from build123d import *

# Parameters (mm, degrees)
MAINBASESKETCH_W         = 7.9
MAINBASESKETCH_H         = 3.2
MAINBASEEXTRUDE_DEPTH    = 7.9
MAINBASESHELL_T          = -1.2
SKETCH171_W              = 5.5
SKETCH171_H              = 1.191135725
BOSS_EXTRUDE23_DEPTH     = 2
CUT_EXTRUDE58_DEPTH      = 12.83470157
CUT_EXTRUDE58_DEPTH_BACK = 12.83470157
SWEEP28_DEPTH            = 3.2
PLAINHALF3_DEPTH         = 2
CUT_EXTRUDE59_DEPTH      = 13.162994561


# Read off the part's stored shape, not the designer's step: Sweep28
with BuildPart() as part:
    # MainBaseSketch → MainBaseExtrude (new, symmetric)
    with BuildSketch(Plane.XY):
        with Locations((4.631967213, 1.6)):
            Rectangle(MAINBASESKETCH_W, MAINBASESKETCH_H)
    extrude(amount=MAINBASEEXTRUDE_DEPTH, both=True)

    # MainBaseShell
    mainbaseshell_openings = [part.faces().sort_by_distance(p)[0] for p in [
        (4.631967213, 0, 0),
    ]]
    offset(amount=MAINBASESHELL_T, openings=mainbaseshell_openings, kind=Kind.INTERSECTION)

    # Sketch171 → Boss-Extrude23 (add)
    with BuildSketch(Plane(origin=(0, 2, 0), x_dir=(-1, 0, 0), z_dir=(0, -1, 0))):
        with Locations((-4.631967213, -0.595567863)):
            Rectangle(SKETCH171_W, SKETCH171_H)
    extrude(amount=BOSS_EXTRUDE23_DEPTH)

    # Sketch173 → Cut-Extrude58 (cut, two sides: drawn at the far end of the back side and taken through both)
    with BuildSketch(Plane(origin=(0, 2, 0), x_dir=(-1, 0, 0), z_dir=(0, -1, 0)).offset(-CUT_EXTRUDE58_DEPTH_BACK)):
        Polygon((-7.381967213, 0), (-8.581967213, 0), (-8.581967213, 7.9), (-0.681967213, 7.9), (-0.681967213, 0), align=None)
    extrude(amount=CUT_EXTRUDE58_DEPTH + CUT_EXTRUDE58_DEPTH_BACK, mode=Mode.SUBTRACT)

    # Sweep28 outline → Sweep28 (add)
    with BuildSketch(Plane(origin=(0, 0, 0), x_dir=(1, 0, 0), z_dir=(0, 1, 0))):
        Polygon((8.581967213, 0), (8.581967213, 8.003016647), (7.381967213, 7.994392876), (0.681967213, 0), align=None)
    extrude(amount=SWEEP28_DEPTH)

    # Sketch174 → PlainHalf3 (cut)
    with BuildSketch(Plane(origin=(0, 0, 0), x_dir=(-1, 0, 0), z_dir=(0, -1, 0))):
        Polygon((-7.381967213, 7.994392876), (-7.381967213, 1.2), (-7.381967213, 0), (-2.361390112, 0), (-2.361390112, 0.487595591), (-2.706140626, 0.958938316), (-1.846183268, 1.587930185), align=None)
    extrude(amount=-PLAINHALF3_DEPTH, mode=Mode.SUBTRACT)

    # Mirror15: part across plane


with BuildPart() as part_1:
    add(part.part)
    add(part.part.mirror(Plane.ZY.offset(-0.681967213)))

    # Sketch178 → Cut-Extrude59 (cut, through all)
    with BuildSketch(Plane(origin=(0, 0, 0), x_dir=(-1, 0, 0), z_dir=(0, -1, 0))):
        Polygon((-8.581967213, -7.9), (-0.681967213, -7.9), (-0.681967213, 0.079862465), (-7.381967213, 7.994392876), (-8.581967213, 8.003016647), align=None)
    extrude(amount=-CUT_EXTRUDE59_DEPTH, mode=Mode.SUBTRACT)


solid = part_1.part
Source: CAD feature listing. Evaluate the final solid. Frame: model axes, mm. A direction names the side the tool comes from. Coordinates: 2 decimals unless noted, no trailing zeros. Write each loop counter-clockwise with the first axis right and the second up, starting at its lowest first coordinate (ties: lowest second). Pieces come first, ordered by that corner, then holes. Notation, with made-up numbers: M 70,63 L 129,63 A14 cw 129,72 Z; hole C 42.5,59.5 d10. An arc over 180 degrees is marked long. Use a Markdown table: item, result.
1) Section D-D, the plane x = -0.75. Output: boundary loops of the cut face in (y, z).
Conclusion:
| item | result |
|---|---|
| outline | M 0,-1.39 L 2,-1.39 L 2,-1.71 L 3.2,-1.71 L 3.2,7.9 L 0,7.9 L 0,6.7 L 2,6.7 L 2,1.19 L 0,1.19 Z |
2) Section C-C, the plane x = -2.5. Output: boundary loops of the cut face in (y, z), then the cut area to 3 significant figures.
Conclusion:
| item | result |
|---|---|
| outline | M 0,0 L 2,0 L 2,-3.8 L 3.2,-3.8 L 3.2,7.9 L 0,7.9 L 0,6.7 L 2,6.7 L 2,1.19 L 0,1.19 Z |
| area | 18.8 mm^2 |
3) Ray query, L1, parallel to Z at x = -5, y = 1.5; L2, parallel to X at y = 1.1, z = 5.25; L3, parallel to X at y = 0.7, z = -6.75. Return the intervals inside material, ascending.
Conclusion:
| item | result |
|---|---|
| L1 | z = 0 to 1.19, 6.7 to 7.9 |
| L2 | x = -7.22 to -6.02, -0.52 to 0.68 |
| L3 | x = -7.22 to -6.02 |
4) Mould query, pull axis Z, two halves, no side actions, for faces 4 (the flat face through (-3, 2, 7.9)), 5 (the flat face through (-3, 2, 4)), 6 (the flat face through (-4, 3.2, 2)). Classes: pulls with the +Z half, pulls with the -Z half, needs draft (parallel to the pull), parting line crosses it, or undercut.
Conclusion:
| item | result |
|---|---|
| face 4 | pulls with the +Z half |
| face 5 | undercut |
| face 6 | needs draft |
5) Reachability of faces 1 (the flat face through (-3, 0, 1)), 2 (the flat face through (-3, 1, 6.7)), 3 (the flat face through (-6.018, 1, -4)) from +Z, -Z, +X, -X, +Y, -Y: full face, straight path, thin tool, end or side. Return the list, or none.
Conclusion:
| item | result |
|---|---|
| face 1 | +Z, -Z, +X, -X, -Y |
| face 2 | -Y |
| face 3 | -Z, -Y |
6) First-contact query: pin 1 Ø1 at (y, z) = (1, -5) entering from +X; pin 2 Ø1.5 at (x, z) = (-4, -4) entering from -Y; pin 3 Ø0.6 at (x, y) = (-2.5, 1) entering from -Z. Flat tips, straight axial feed; report the tip coordinate or a pass-through.
Conclusion:
| item | result |
|---|---|
| pin 1 | stops at x = -6.02 |
| pin 2 | stops at y = 2 |
| pin 3 | stops at z = 0 |
7) Section B-B, the plane z = 3.5. Output: boundary loops of the cut face in (x, y), then the cut area to 3 significant figures.
Conclusion:
| item | result |
|---|---|
| outline | M -7.22,0 L -6.02,0 L -6.02,2 L -0.52,2 L -0.52,0 L 0.68,0 L 0.68,3.2 L -7.22,3.2 Z |
| area | 14.3 mm^2 |
8) Section A-A, the plane y = 1.85. Output: boundary loops of the cut face in (x, z).
Conclusion:
| item | result |
|---|---|
| outline | M -7.22,-8 L -6.02,-7.99 L -6.02,0 L -1,0 L -1,-0.49 L -1.34,-0.96 L -0.59,-1.51 L 0.68,0 L 0.68,7.9 L -7.22,7.9 Z; hole M -6.02,1.19 L -0.52,1.19 L -0.52,6.7 L -6.02,6.7 Z |
